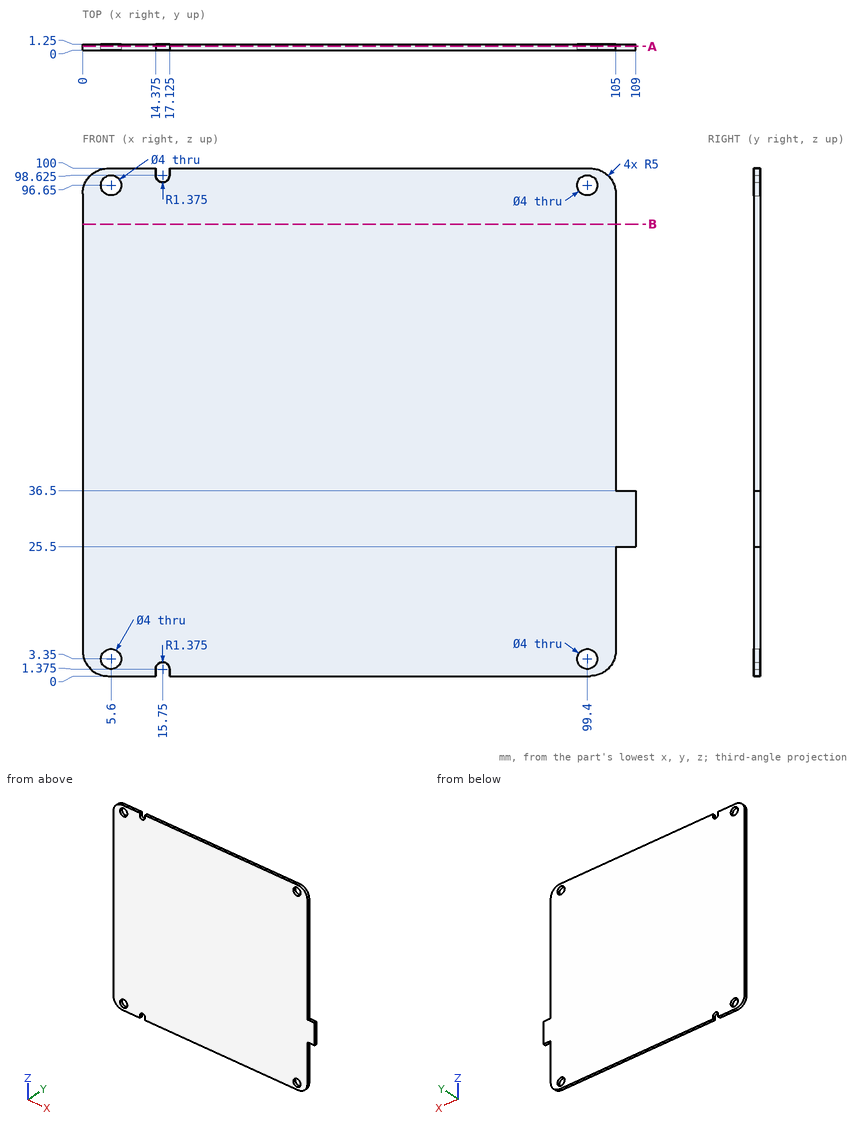
Could you check a few things on this drawing? It's one solid part, dimensions in mm from its lowest x, y, z. Coordinates: 2 decimals unless noted, no trailing zeros. Write each loop counter-clockwise with the first axis right and the second up, starting at its lowest first coordinate (ties: lowest second). Pieces come first, ordered by that corner, then holes. Notation, with made-up numbers: M 7.5,68 L 63.5,68 A22 cw 63.5,97 Z; hole C 24.25,-10.75 d5. An arc over 180 degrees is marked long. Answer as CSV lines item,"result". Start each with the question number.
Q1. Suppose I cut it at B-B, the plane z = 89. List the corners of the cut face in (x, y) for me, then the cut area to 3 significant figures.
Q2. Will these pins go through, and if not, where does the flat tip stop? pin 1 Ø6.5 at (x, z) = (99.4, 3.35) entering from +Y; pin 2 Ø0.6 at (y, z) = (1, 0.5) entering from +X; pin 3 Ø0.6 at (y, z) = (1, 99) entering from +X; pin 4 Ø3.5 at (x, z) = (99.4, 96.65) entering from -Y.
Q3. I need wall thicknesses on probe 1 along Z at (x, y) = (99.4, 0.45); probe 2 along X at (y, z) = (0.5, 96.65); probe 3 along X at (y, z) = (1.2, 53.5). Which ranges of each line are inside material? Lowest first, please. Write a range as [from, to].
Q4. Suppose I cut it at A-A, the plane y = 0.8. List the corners of the cut face in (x, z) for me (3 decimals).
Entries:
1,outline,"M 0,0 L 105,0 L 105,1.25 L 0,1.25 Z"
1,area,"131 mm²"
2,pin 1,"stops at y = 1.25"
2,pin 2,"stops at x = 102.71"
2,pin 3,"stops at x = 103.36"
2,pin 4,"passes through"
3,probe 1,"z = [0, 1.35], [5.35, 94.65], [98.65, 100]"
3,probe 2,"x = [0.28, 3.6], [7.6, 97.4], [101.4, 104.72]"
3,probe 3,"x = [0, 105]"
4,outline,"M 0,5 A5 ccw 5,0 L 14.375,0 L 14.375,1.375 A1.375 cw 17.125,1.375 L 17.125,0 L 100,0 A5 ccw 105,5 L 105,25.5 L 109,25.5 L 109,36.5 L 105,36.5 L 105,95 A5 ccw 100,100 L 17.125,100 L 17.125,98.625 A1.375 cw 14.375,98.625 L 14.375,100 L 5,100 A5 ccw 0,95 Z; hole C 5.6,3.35 d4; hole C 5.6,96.65 d4; hole C 99.4,3.35 d4; hole C 99.4,96.65 d4"
